The figure shows three views and two pictorial views of one solid part (mm, origin at its lowest corner). Answer the questions. A direction names the side the tool comes from. Coordinates: 2 decimals unless noted, no trailing zeros. Order: outer loops, then holes, each group sorted by start corner. A loop starts at its lowest first (then second) coordinate and runs counter-clockwise, first axis right, second up. Notation, with made-up numbers: (47.5, -12.75) -> (74.5, -12.75) arc R24 ccw to (74.5, 5.25) -> close; hole circle Ø8 at (32.25, -16.75). An arc over 180 degrees is marked (long way). Use one line per item in the form item = value.
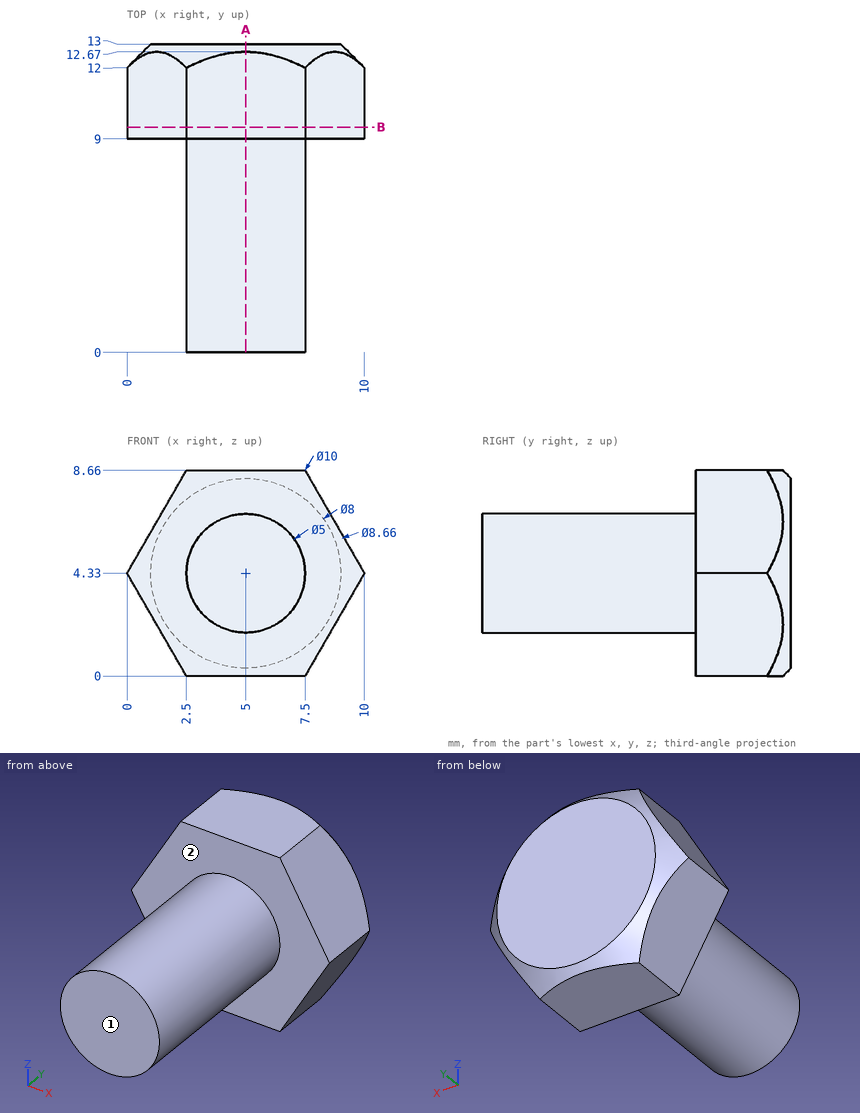
(1) Section A-A on x = 5 is taken. Write down the section's boundary in (y, z).
Data:
outline = (0, 1.83) -> (9, 1.83) -> (9, 0) -> (12.67, 0) -> (13, 0.33) -> (13, 8.33) -> (12.67, 8.66) -> (9, 8.66) -> (9, 6.83) -> (0, 6.83) -> close
(2) Each of these flat-tipped pins is pushed along its axis until it touches: P1, Ø5, axis at y = 4, z = 1, coming from the -X side; P2, Ø3, axis at y = 4.5, z = 2, coming from the +X side; P3, Ø5, axis at x = 5.5, y = 7, coming from the -Z side; P4, Ø2, axis at y = 10, z = 5.5, coming from the -X side. Where does it stop, or does it pass through?
Data:
P1 = 2.64
P2 = 7.36
P3 = 0
P4 = 0.1
(3) Section B-B on y = 9.5 is taken. Write down the section's boundary in (x, z).
Data:
outline = (0, 4.33) -> (2.5, 0) -> (7.5, 0) -> (10, 4.33) -> (7.5, 8.66) -> (2.5, 8.66) -> close
(4) Straight lines are drawn through the part: line 1 along Y through (x, z) = (3, 1); line 2 along X through (y, z) = (10, 3); line 3 along Z through (x, y) = (4, 1.75). For each, find the intervals that lie inside material, in ascending order.
Data:
line_1 = 9 to 13
line_2 = 0.77 to 9.23
line_3 = 2.04 to 6.62
(5) Which of the six approach directions +Z, -Z, +X, -X, +Y, -Y give full straight-line access (tool end or side, diameter ignored) to the marked faces 1 and 2?
Data:
face_1 = +Z, -Z, +X, -X, -Y
face_2 = -Y
